Source: CAD feature listing. Evaluate the final solid. Frame: model axes, mm. A direction names the side the tool comes from. Round coordinates to 2 decimals unless told otherwise and drop trailing zeros. Order: outer loops, then holes, each group sorted by start corner. A loop starts at its lowest first (then second) coordinate and runs counter-clockwise, first axis right, second up. Notation, with made-up numbers: (22, 5) - (55, 5) arc R17 cw to (55, 14) - close; hole circle Ø9 at (13.25, -31.5). An arc over 180 degrees is marked (long way). Use one line per item in the form item = value. Start each with the question number.
Q1. Cut plane B-B, the plane y = 5. Return the cut outline in (x, z).
Q2. Set-up query: faces 1 (the flat face through (8, 0, 6)), 2 (the flat face through (0, -1, 2)). Return all of +Z, -Z, +X, -X, +Y, -Y with unobstructed straight access to the full face (end or side cutting, diameter ignored); none if empty.
Q3. Ray query, line 1 (X direction, y = -2.75, z = 7); line 2 (Z direction, x = 1.5, y = 4.25); line 3 (Y direction, x = 5, z = 8). Return the intervals inside material, ascending. Write a range as [from, to].
Q4. Pin query (flat end, axial travel): pin 1 Ø2.5 at (x, z) = (0, 5) entering from -Y. Return the tip coordinate at first contact, or that it passes through.
Q5. Cut plane A-A, the plane z = 8.75. Return the cut outline in (x, y).
Q6. Cut plane C-C, the plane x = 1. Return the cut outline in (y, z), and give its area (3 significant figures).
Autodesk Inventor part; units mm, degrees
ref_plane "YZ Plane" through (0, 0, 0) normal (1, 0, 0) x (0, 1, 0)
ref_plane "XZ Plane" through (0, 0, 0) normal (0, 1, 0) x (-1, 0, 0)
ref_plane "XY Plane" through (0, 0, 0) normal (0, 0, 1) x (1, 0, 0)
sketch "Skizze1" plane through (0, 0, 0) normal (0, 0, 1) x (1, 0, 0)
  line L0 (-8, -7.5) -> (8, -7.5)
  line L1 (8, -7.5) -> (8, 7.5)
  line L2 (8, 7.5) -> (-8, 7.5)
  line L3 (-8, 7.5) -> (-8, -7.5)
  line L4 (-8, -7.5) -> (8, 7.5) construction
  line L5 (8, -7.5) -> (-8, 7.5) construction
  point P0 (0, 0)
  dimension "d0" = 16
  dimension "d1" = 15
extrude "Extrusion1" add sketch "Skizze1" along normal blind 13
shell "Wandstärke1" thickness 2 removed faces 1 at (-2.6667, -7.5, 4.3333)
properties part number "RJ45-Buchse" material "Stahl, verchromt"
Completed:
q1.outline = (-8, 0) - (8, 0) - (8, 13) - (-8, 13) - close; hole (-6, 2) - (6, 2) - (6, 11) - (-6, 11) - close
q2.face_1 = +Z, -Z, +X, +Y, -Y
q2.face_2 = -Y
q3.line_1 = [-8, -6], [6, 8]
q3.line_2 = [0, 2], [11, 13]
q3.line_3 = [5.5, 7.5]
q4.pin_1 = 5.5
q5.outline = (-8, -7.5) - (-6, -7.5) - (-6, 5.5) - (6, 5.5) - (6, -7.5) - (8, -7.5) - (8, 7.5) - (-8, 7.5) - close
q6.outline = (-7.5, 0) - (7.5, 0) - (7.5, 13) - (-7.5, 13) - (-7.5, 11) - (5.5, 11) - (5.5, 2) - (-7.5, 2) - close
q6.area = 78.0 mm2
